Geometry check sheet. Reference: the model listing, model coordinates, mm. Face numbers are marked on the shaded views. A direction names the side the tool comes from. Give positions to 0.01 mm unless a question says otherwise; leave off trailing zeros. Order: outer loops, then holes, each group sorted by start corner. A loop starts at its lowest first (then second) coordinate and runs counter-clockwise, first axis right, second up. Notation, with made-up numbers: M 2.25,4 L 22.25,4 A10 ccw 22.25,8 Z; hole C -11.75,10 d6. An arc over 180 degrees is marked long. Use CSV: the item, a comma, the result in double quotes. Start each with the question number.
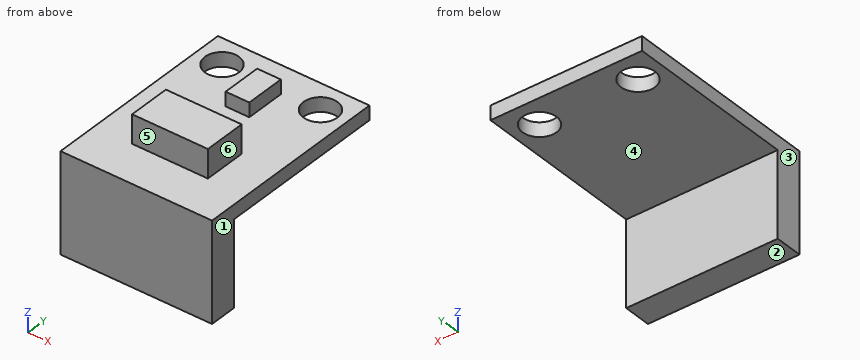
from build123d import *

# Parameters (mm, degrees)
SKETCH1_W           = 16
SKETCH1_H           = 21
SKETCH1_R           = 1.8
BOSS_EXTRUDE1_DEPTH = 1.5
SKETCH2_W           = 2.5
SKETCH2_H           = 4.2
BOSS_EXTRUDE2_DEPTH = 1.5
SKETCH3_W           = 8
SKETCH3_H           = 4.5
BOSS_EXTRUDE3_DEPTH = 3
SKETCH4_W           = 16
SKETCH4_H           = 2.9
BOSS_EXTRUDE4_DEPTH = 9


with BuildPart() as part:
    # Sketch1 → Boss-Extrude1 (new body)
    with BuildSketch(Plane.XY):
        Rectangle(SKETCH1_W, SKETCH1_H)
        with Locations((-5.2, 7.5)):
            Circle(SKETCH1_R, mode=Mode.SUBTRACT)
        with Locations(Location((5.2, 7.5, 0), (0, 0, 180))):
            Circle(SKETCH1_R, mode=Mode.SUBTRACT)
    extrude(amount=BOSS_EXTRUDE1_DEPTH)

    # Sketch2 → Boss-Extrude2 (add)
    with BuildSketch(Plane.XY.offset(1.5)):
        with Locations((0, 5.1)):
            Rectangle(SKETCH2_W, SKETCH2_H)
    extrude(amount=BOSS_EXTRUDE2_DEPTH)

    # Sketch3 → Boss-Extrude3 (add)
    with BuildSketch(Plane.XY.offset(1.5)):
        with Locations((0, -3.75)):
            Rectangle(SKETCH3_W, SKETCH3_H)
    extrude(amount=BOSS_EXTRUDE3_DEPTH)

    # Sketch4 → Boss-Extrude4 (add)
    with BuildSketch(Plane(origin=(0, 0, 0), x_dir=(-1, 0, 0), z_dir=(0, 0, -1))):
        with Locations((0, -9.05)):
            Rectangle(SKETCH4_W, SKETCH4_H)
    extrude(amount=BOSS_EXTRUDE4_DEPTH)


solid = part.part
(1) Sectioned sample at B-B on y = 7.5. Record the cut outline in (x, z).
(2) Go/stop test with flat-tipped pins: P1, Ø4, axis at x = 6.5, y = 2.5, coming from the +Z side; P2, Ø0.8, axis at x = 0, y = 5.5, coming from the +Z side; P3, Ø0.8, axis at x = 0, z = 2, coming from the -Y side; P4, Ø3.5, axis at x = -1.5, z = 3, coming from the -Y side. Record where each tip stops, or that it passes through.
(3) Draft check along X on the marked faces 1, 2 and 3. Enter one of: +X half, -X half, draft (parallel to the pull), parting line (faces both ways), or undercut.
(4) Sectioned sample at C-C on y = 4. Record the cut outline in (x, z).
(5) Access from +Z, -Z, +X, -X, +Y, -Y to the whole of each face (thin tool, end or side, straight path). Record for the marked faces 4, 5 and 6.
(6) Sectioned sample at A-A on x = -5.2. Record the cut outline in (y, z), then the cut area to 3 significant figures.
(7) Sectioned sample at D-D on z = -6. Record the cut outline in (x, y), then the cut area to 3 significant figures.
(8) Thickness scan on line 1 (Y direction, x = -5.2, z = 1.2); line 2 (Y direction, x = 1.75, z = -1.75); line 3 (Z direction, x = 0.25, y = 4.25). Record the ranges inside material, lowest first.
Responses:
1,outline,"M -8,0 L -7,0 L -7,1.5 L -8,1.5 Z; M -3.4,0 L 3.4,0 L 3.4,1.5 L -3.4,1.5 Z; M 7,0 L 8,0 L 8,1.5 L 7,1.5 Z"
2,P1,"z = 1.5"
2,P2,"z = 3"
2,P3,"y = -6"
2,P4,"y = -10.5"
3,face 1,"+X half"
3,face 2,"draft"
3,face 3,"-X half"
4,outline,"M -8,0 L 8,0 L 8,1.5 L 1.25,1.5 L 1.25,3 L -1.25,3 L -1.25,1.5 L -8,1.5 Z"
5,face 4,"-Z, +X, -X, +Y"
5,face 5,"+Z, +X, -X, -Y"
5,face 6,"+Z, +X, +Y, -Y"
6,outline,"M -10.5,-9 L -7.6,-9 L -7.6,0 L 5.7,0 L 5.7,1.5 L -10.5,1.5 Z; M 9.3,0 L 10.5,0 L 10.5,1.5 L 9.3,1.5 Z"
6,area,"52.2 mm2"
7,outline,"M -8,-10.5 L 8,-10.5 L 8,-7.6 L -8,-7.6 Z"
7,area,"46.4 mm2"
8,line 1,"-10.5 to 5.7, 9.3 to 10.5"
8,line 2,"-10.5 to -7.6"
8,line 3,"0 to 3"
